from build123d import *

# Parameters (mm, degrees)
SKETCH1_W             = 100
SKETCH1_H             = 65.25
SKETCH1_W_2           = 96
SKETCH1_H_2           = 62.64
BOSS_EXTRUDE1_DEPTH   = 40
CUT_EXTRUDE1_REACH    = 93.42
SKETCH2_R             = 2
SKETCH3_R             = 4
SKETCH3_R_2           = 1.5
BOSS_EXTRUDE2_DEPTH   = 2
BOSS_EXTRUDE2_2_DEPTH = 2
BOSS_EXTRUDE4_DEPTH   = 2
FILLET1_R             = 4


with BuildPart() as part:
    # Sketch1 → Boss-Extrude1 (new body)
    with BuildSketch(Plane(origin=(0, 0, 0), x_dir=(1, 0, 0), z_dir=(0, 1, 0))):
        Rectangle(SKETCH1_W, SKETCH1_H)
        Rectangle(SKETCH1_W_2, SKETCH1_H_2, mode=Mode.SUBTRACT)
    extrude(amount=BOSS_EXTRUDE1_DEPTH)

    # Sketch2 → Cut-Extrude1 (cut, up to next)
    with BuildSketch(Plane.XY.offset(32.625), mode=Mode.PRIVATE) as cut_extrude1_sk1:
        with Locations((-43, 15)):
            Circle(SKETCH2_R)
    cut_extrude1_tool1 = extrude(cut_extrude1_sk1.sketch, amount=-CUT_EXTRUDE1_REACH, mode=Mode.PRIVATE) & part.part
    # Sketch2 → Cut-Extrude1 (cut, up to next)
    with BuildSketch(Plane.XY.offset(32.625), mode=Mode.PRIVATE) as cut_extrude1_sk2:
        with Locations((-43, 30)):
            Circle(SKETCH2_R)
    cut_extrude1_tool2 = extrude(cut_extrude1_sk2.sketch, amount=-CUT_EXTRUDE1_REACH, mode=Mode.PRIVATE) & part.part
    # Sketch2 → Cut-Extrude1 (cut, up to next)
    with BuildSketch(Plane.XY.offset(32.625), mode=Mode.PRIVATE) as cut_extrude1_sk3:
        with Locations((43, 30)):
            Circle(SKETCH2_R)
    cut_extrude1_tool3 = extrude(cut_extrude1_sk3.sketch, amount=-CUT_EXTRUDE1_REACH, mode=Mode.PRIVATE) & part.part
    # Sketch2 → Cut-Extrude1 (cut, up to next)
    with BuildSketch(Plane.XY.offset(32.625), mode=Mode.PRIVATE) as cut_extrude1_sk4:
        with Locations((43, 15)):
            Circle(SKETCH2_R)
    cut_extrude1_tool4 = extrude(cut_extrude1_sk4.sketch, amount=-CUT_EXTRUDE1_REACH, mode=Mode.PRIVATE) & part.part
    add(cut_extrude1_tool1.solids().sort_by_distance((-43, 15, 32.625))[0], mode=Mode.SUBTRACT)
    add(cut_extrude1_tool2.solids().sort_by_distance((-43, 30, 32.625))[0], mode=Mode.SUBTRACT)
    add(cut_extrude1_tool3.solids().sort_by_distance((43, 30, 32.625))[0], mode=Mode.SUBTRACT)
    add(cut_extrude1_tool4.solids().sort_by_distance((43, 15, 32.625))[0], mode=Mode.SUBTRACT)



with BuildPart() as body_2:
    # Sketch3 → Boss-Extrude2 (new body)
    with BuildSketch(Plane(origin=(0, 40, 0), x_dir=(1, 0, 0), z_dir=(0, 1, 0))):
        with Locations(Location((-24, -5.32, 0), (0, 0, 270))):
            Circle(SKETCH3_R)
        with Locations(Location((-24, -5.32, 0), (0, 0, 270))):
            Circle(SKETCH3_R_2, mode=Mode.SUBTRACT)
    extrude(amount=-BOSS_EXTRUDE2_DEPTH)


with BuildPart() as body_3:
    # Sketch3 → Boss-Extrude2 2 (new body)
    with BuildSketch(Plane(origin=(0, 40, 0), x_dir=(1, 0, 0), z_dir=(0, 1, 0))):
        with Locations(Location((24, -5.32, 0), (0, 0, 270))):
            Circle(SKETCH3_R)
        with Locations(Location((24, -5.32, 0), (0, 0, 270))):
            Circle(SKETCH3_R_2, mode=Mode.SUBTRACT)
    extrude(amount=-BOSS_EXTRUDE2_2_DEPTH)


with BuildPart() as part_1:
    add(part.part)

    add(body_2.part)  # Boss-Extrude4 merges body 2

    add(body_3.part)  # Boss-Extrude4 merges body 3
    # Sketch4 → Boss-Extrude4 (add)
    with BuildSketch(Plane(origin=(0, 40, 0), x_dir=(-1, 0, 0), z_dir=(0, -1, 0))):
        with BuildLine():
            Line((-24.225075601, -1.326337399), (-45.609139399, 31.32))
            Line((-45.609139399, 31.32), (-48, 31.32))
            Line((-48, 31.32), (-48, 27.669952816))
            Line((-48, 27.669952816), (-27.571151067, -3.518089888))
            ThreePointArc((-27.571151067, -3.518089888), (-26.191752489, -1.973924534), (-24.225075601, -1.326337399))
        make_face()
        with BuildLine():
            Line((-27.819238089, -6.508873594), (-48, -28.371365665))
            Line((-48, -28.371365665), (-48, -31.32))
            Line((-48, -31.32), (-45.27818369, -31.32))
            Line((-45.27818369, -31.32), (-24.88002431, -9.221994005))
            ThreePointArc((-24.88002431, -9.221994005), (-26.713120411, -8.259213779), (-27.819238089, -6.508873594))
        make_face()
        with BuildLine():
            Line((24.225075601, -1.326337399), (45.609139399, 31.32))
            Line((45.609139399, 31.32), (48, 31.32))
            Line((48, 31.32), (48, 27.669952816))
            Line((48, 27.669952816), (27.571151067, -3.518089888))
            ThreePointArc((27.571151067, -3.518089888), (26.191752489, -1.973924534), (24.225075601, -1.326337399))
        make_face()
        with BuildLine():
            Line((48, -28.371365665), (48, -31.32))
            Line((48, -31.32), (45.27818369, -31.32))
            Line((45.27818369, -31.32), (24.88002431, -9.221994005))
            ThreePointArc((24.88002431, -9.221994005), (26.713120411, -8.259213779), (27.819238089, -6.508873594))
            Line((27.819238089, -6.508873594), (48, -28.371365665))
        make_face()
    extrude(amount=BOSS_EXTRUDE4_DEPTH)

    # Fillet1
    fillet1_edges = [part_1.edges().sort_by_distance(p)[0] for p in [
        (-24.88002431, 39, 9.221994005),
        (-27.819238089, 39, 6.508873594),
        (-48, 39, 28.371365665),
        (-45.27818369, 39, 31.32),
        (45.609139399, 39, -31.32),
        (24.225075601, 39, 1.326337399),
        (27.571151067, 39, 3.518089888),
        (48, 39, -27.669952816),
        (-27.571151067, 39, 3.518089888),
        (-24.225075601, 39, 1.326337399),
        (-45.609139399, 39, -31.32),
        (-48, 39, -27.669952816),
        (48, 39, 28.371365665),
        (27.819238089, 39, 6.508873594),
        (24.88002431, 39, 9.221994005),
        (45.27818369, 39, 31.32),
    ]]
    fillet(fillet1_edges, radius=FILLET1_R)


solid = part_1.part
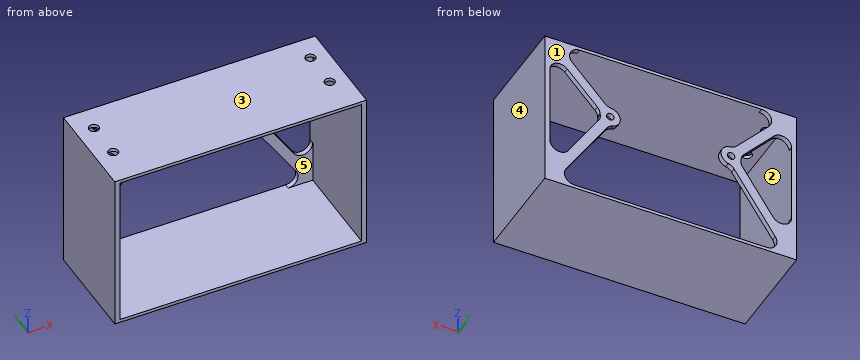
For this review, take the finished solid that the model builds, in its own axes (mm). Face numbers are marked on the shaded views. A direction names the side the tool comes from. Round coordinates to 2 decimals unless told otherwise and drop trailing zeros. Order: outer loops, then holes, each group sorted by start corner. A loop starts at its lowest first (then second) coordinate and runs counter-clockwise, first axis right, second up. Notation, with made-up numbers: M -6,15 L -1,15 A25 cw -1,54 Z; hole C 83,-16.5 d7. An arc over 180 degrees is marked long. Use a Markdown table: item, result. Add a question column.
Item 1: Add section C-C, the plane z = 13.5. Give the boundary of the cut face in (x, y), then the cut area to 3 significant figures.
Item 2: Insertion check: pin 1 (6.5 mm diameter, centred on x = 43, y = 30, fed in from +Z) (3 decimals); pin 2 (1.8 mm diameter, centred on x = 24, z = 5.32, fed in from +Y). Each pin has a flat end and moves straight along its axis. Give the tip position at first contact, or say it passes through.
Item 3: Add section A-A, the plane y = 15. Give the boundary of the cut face in (x, z) (3 decimals).
Item 4: To check wall thickness, follow line 1 along Y through (x, z) = (43, 31.85); line 2 along Z through (x, y) = (45, 13) (3 decimals); line 3 along X through (y, z) = (3.5, -12.5). State the ranges of each line that lie inside material, in increasing order.
Item 5: Mouldability with a two-part tool opening along Z and no side actions: class the marked faces 1, 2 and 3 as released by +Z, released by -Z, zero draft, split by the parting line, or undercut.
Item 6: Add section B-B, the plane x = -34. Give the boundary of the cut face in (y, z) (3 decimals).
Item 7: Tool access review of the marked faces 4 and 5: name each direction out of +Z, -Z, +X, -X, +Y, -Y from which nothing blocks a thin tool from reaching the whole face with its end or side.
Geometry results:
| question | item | result |
|---|---|---|
| 1 | outline | M -50,0 L -48,0 L -48,40 L -50,40 Z; M -34.27,38 L -28.83,38 L -28.83,40 L -34.27,40 Z; M 28.83,38 L 34.27,38 L 34.27,40 L 28.83,40 Z; M 48,0 L 50,0 L 50,40 L 48,40 Z |
| 1 | area | 182 mm² |
| 2 | pin 1 | stops at z = 32.625 |
| 2 | pin 2 | passes through |
| 3 | outline | M -50,-32.625 L 50,-32.625 L 50,32.625 L 45,32.625 L 45,31.32 L 48,31.32 L 48,-31.32 L -48,-31.32 L -48,31.32 L -45,31.32 L -45,32.625 L -50,32.625 Z; M -41,31.32 L 41,31.32 L 41,32.625 L -41,32.625 Z |
| 4 | line 1 | y = 0 to 13, 17 to 28, 32 to 40 |
| 4 | line 2 | z = -32.625 to -31.32, 31.32 to 32.625 |
| 4 | line 3 | x = -50 to -48, 48 to 50 |
| 5 | face 1 | zero draft |
| 5 | face 2 | undercut |
| 5 | face 3 | released by +Z |
| 6 | outline | M 0,-32.625 L 40,-32.625 L 40,-31.32 L 0,-31.32 Z; M 0,31.32 L 40,31.32 L 40,32.625 L 0,32.625 Z; M 38,-13.597 L 40,-13.597 L 40,-6.297 L 38,-6.297 Z; M 38,13.205 L 40,13.205 L 40,19.102 L 38,19.102 Z |
| 7 | face 4 | +Z, -Z, +X, +Y, -Y |
| 7 | face 5 | -Y |
